```python
from build123d import *

# Parameters (mm, degrees)
SKETCH_1_W      = 21
SKETCH_1_H      = 16
SKETCH_1_R      = 1.6
EXTRUDE_1_DEPTH = 2
EXTRUDE_2_DEPTH = 21


with BuildPart() as part:
    # 草图1 → 凸台-拉伸1 (new body)
    with BuildSketch(Plane(origin=(0, 0, 0), x_dir=(1, 0, 0), z_dir=(0, 1, 0))):
        with Locations((10.5, 8)):
            Rectangle(SKETCH_1_W, SKETCH_1_H)
        with Locations(Location((18.5, 2, 0), (0, 0, 270))):
            Circle(SKETCH_1_R, mode=Mode.SUBTRACT)
        with Locations(Location((2.5, 2, 0), (0, 0, 90))):
            Circle(SKETCH_1_R, mode=Mode.SUBTRACT)
    extrude(amount=EXTRUDE_1_DEPTH)

    # 草图3 → 凸台-拉伸2 (add)
    with BuildSketch(Plane(origin=(21, 0, 0), x_dir=(0, 0, -1), z_dir=(1, 0, 0))):
        Polygon((16, 2), (14, 2), (14, 7), (22, 7), (22, 5.5), (16, 5.5), align=None)
    extrude(amount=-EXTRUDE_2_DEPTH)


solid = part.part
```
The listing builds one solid part. Answer for the finished solid, in the listing's coordinates (mm). A direction names the side the tool comes from. Coordinates: 2 decimals unless noted, no trailing zeros. Write each loop counter-clockwise with the first axis right and the second up, starting at its lowest first coordinate (ties: lowest second). Pieces come first, ordered by that corner, then holes. Notation, with made-up numbers: (76.5, -33) - (82.5, -33) arc R22 ccw to (82.5, -20) - close; hole circle Ø6 at (-13.75, 6.5). An arc over 180 degrees is marked (long way). Return JSON: item names as keys, results as strings. Group by question number.
1. Determine the mould class of faces 1 (the flat face through (11, 3, -16)), 2 (the cylindrical face through (20.086, 0.986, -2.208)), 3 (the flat face through (11, 5.5, -19)) for opening direction Z: released by +Z, released by -Z, zero draft, split by the parting line, or undercut.
2. A cutting plane is placed at A-A, the plane z = -2. Determine the outline of the cut face in (x, y), plus the area to 3 significant figures.
3. Straight lines are drawn through the part: L1, parallel to X at y = 0.75, z = -2; L2, parallel to Z at x = 14.75, y = 3.5; L3, parallel to X at y = 1.25, z = -1.25. For each, find the intervals that lie inside material, in ascending order.
4. A cutting plane is placed at B-B, the plane x = 3.75. Determine the outline of the cut face in (y, z), plus the area to 3 significant figures.
5. Which of the six approach directions +Z, -Z, +X, -X, +Y, -Y give full straight-line access (tool end or side, diameter ignored) to faces 4 (the flat face through (11, 4, -14)), 5 (the flat face through (0, 1.7, -11.1))?
6. A cutting plane is placed at C-C, the plane x = 13. Determine the outline of the cut face in (y, z), plus the area to 3 significant figures.
7. A cutting plane is placed at D-D, the plane y = 5.25. Determine the outline of the cut face in (x, z), plus the area to 3 significant figures.
8. Given pin 1 (1 mm diameter, centred on x = 12.5, y = 5, fed in from +Z); pin 2 (5 mm diameter, centred on x = 12, z = -20, fed in from -Y); pin 3 (1.6 mm diameter, centred on x = 7, y = 2, fed in from -Z), each flat-ended and moving along its own axis, determine where each tip first touches the part or whether it passes through.
Ans:
{
 "1": {"face 1": "released by -Z", "face 2": "undercut", "face 3": "zero draft"},
 "2": {"outline": "(0, 0) - (0.9, 0) - (0.9, 2) - (0, 2) - close; (4.1, 0) - (16.9, 0) - (16.9, 2) - (4.1, 2) - close; (20.1, 0) - (21, 0) - (21, 2) - (20.1, 2) - close", "area": "29.2 mm²"},
 "3": {"L1": "0 to 0.9, 4.1 to 16.9, 20.1 to 21", "L2": "-16 to -14", "L3": "0 to 1.09, 3.91 to 17.09, 19.91 to 21"},
 "4": {"outline": "(0, -16) - (5.5, -16) - (5.5, -22) - (7, -22) - (7, -14) - (2, -14) - (2, -3) - (0, -3) - close; (0, -1) - (2, -1) - (2, 0) - (0, 0) - close", "area": "47.0 mm²"},
 "5": {"face 4": "+Z, +X, -X, +Y", "face 5": "+Z, -Z, -X, +Y, -Y"},
 "6": {"outline": "(0, -16) - (5.5, -16) - (5.5, -22) - (7, -22) - (7, -14) - (2, -14) - (2, 0) - (0, 0) - close", "area": "51.0 mm²"},
 "7": {"outline": "(0, -16) - (21, -16) - (21, -14) - (0, -14) - close", "area": "42.0 mm²"},
 "8": {"pin 1": "z = -14", "pin 2": "y = 5.5", "pin 3": "z = -16"}
}
